Source: CAD feature listing. Evaluate the final solid. Frame: model axes, mm. Face numbers are marked on the shaded views. A direction names the side the tool comes from. Give positions to 0.01 mm unless a question says otherwise; leave off trailing zeros. Loops run counter-clockwise (first coordinate to the right, second up) from the corner with the lowest first, then second, coordinate; pieces in that order, holes last. Notation, with made-up numbers: (34.25, 76) -> (61.25, 76) arc R23 cw to (61.25, 113) -> close; hole circle Ø3 at (-30.75, 31). An arc over 180 degrees is marked (long way). Put each result on its own line as item: value.
```python
from build123d import *

# Parameters (mm, degrees)
SKETCH1_R               = 17.5
SKETCH1_R_2             = 12.5
BOSS_EXTRUDE1_DEPTH     = 152.4
SKETCH2_R               = 19.05
SKETCH2_R_2             = 17.5
BOSS_EXTRUDE2_DEPTH     = 8
SKETCH4_R               = 17.5
SKETCH4_R_2             = 16
CUT_EXTRUDE2_DEPTH      = 2
FILLET1_R               = 0.4064
CUT_EXTRUDE3_DEPTH      = 155.762931608
CUT_EXTRUDE3_DEPTH_BACK = 155.762931608
SKETCH8_W               = 25.4
SKETCH8_H               = 3.175
FILLET2_R               = 3.175
CUT_EXTRUDE4_REACH      = 156.763
CUT_EXTRUDE4_END_RADIUS = 17.5


with BuildPart() as part:
    # Sketch1 → Boss-Extrude1 (new, symmetric)
    with BuildSketch(Plane(origin=(0, 0, 0), x_dir=(0, 0, -1), z_dir=(1, 0, 0))):
        with Locations(Location((0, 0, 0), (0, 0, 180))):
            Circle(SKETCH1_R)
        with Locations(Location((0, 0, 0), (0, 0, 180))):
            Circle(SKETCH1_R_2, mode=Mode.SUBTRACT)
    extrude(amount=BOSS_EXTRUDE1_DEPTH, both=True)

    # Sketch2 → Boss-Extrude2 (add)
    with BuildSketch(Plane.ZY.offset(-92.4)):
        Circle(SKETCH2_R)
        Circle(SKETCH2_R_2, mode=Mode.SUBTRACT)
    extrude(amount=BOSS_EXTRUDE2_DEPTH)

    # Sketch4 → Cut-Extrude2 (cut)
    with BuildSketch(Plane(origin=(133.52, 0, 0), x_dir=(0, 0, -1), z_dir=(1, 0, 0))):
        with Locations(Location((0, 0, 0), (0, 0, 180))):
            Circle(SKETCH4_R)
        Circle(SKETCH4_R_2, mode=Mode.SUBTRACT)
    extrude(amount=-CUT_EXTRUDE2_DEPTH, mode=Mode.SUBTRACT)

    # Fillet1
    fillet1_edges = [part.edges().sort_by_distance(p)[0] for p in [
        (131.52, 0, 16),
        (133.52, 0, 16),
    ]]
    fillet(fillet1_edges, radius=FILLET1_R)

    # Sketch8 → Cut-Extrude3 (cut, two sides: drawn at the far end of the back side and taken through both)
    with BuildSketch(Plane.XY.offset(-CUT_EXTRUDE3_DEPTH_BACK)):
        with Locations((36.7, 17.4625)):
            Rectangle(SKETCH8_W, SKETCH8_H)
        with Locations((36.7, -17.4625)):
            Rectangle(SKETCH8_W, SKETCH8_H)
    extrude(amount=CUT_EXTRUDE3_DEPTH + CUT_EXTRUDE3_DEPTH_BACK, mode=Mode.SUBTRACT)

    # Fillet2
    # the kernel refuses this fillet: 3.175 mm, written as the material it adds along each edge
    with BuildSketch(Plane(origin=(49.4, -15.875, 15.301899161), x_dir=(-1, 0, 0), z_dir=(0, 0, -1))) as fillet2_piece_1_section:
        with BuildLine():
            CenterArc((FILLET2_R, -FILLET2_R), FILLET2_R, 90, 90)
            Line((0, -FILLET2_R), (0, 0))
            Line((0, 0), (FILLET2_R, 0))
        make_face()
    fillet2_piece_1 = extrude(amount=30.603798322, mode=Mode.PRIVATE)
    fillet2_piece_1 = fillet2_piece_1 & Plane(origin=(48.505622485, 0, 0), x_dir=(0, 0, 1), z_dir=(1, 0, 0)) * Cylinder(17.5, 74, mode=Mode.PRIVATE)
    add(fillet2_piece_1)
    with BuildSketch(Plane(origin=(24, -15.875, -15.301899161), x_dir=(1, 0, 0), z_dir=(0, 0, 1))) as fillet2_piece_2_section:
        with BuildLine():
            CenterArc((FILLET2_R, -FILLET2_R), FILLET2_R, 90, 90)
            Line((0, -FILLET2_R), (0, 0))
            Line((0, 0), (FILLET2_R, 0))
        make_face()
    fillet2_piece_2 = extrude(amount=30.603798322, mode=Mode.PRIVATE)
    fillet2_piece_2 = fillet2_piece_2 & Plane(origin=(24.894377515, 0, 0), x_dir=(0, 0, 1), z_dir=(1, 0, 0)) * Cylinder(17.5, 74, mode=Mode.PRIVATE)
    add(fillet2_piece_2)
    with BuildSketch(Plane(origin=(49.4, 15.875, 15.301899161), x_dir=(-1, 0, 0), z_dir=(0, 0, -1))) as fillet2_piece_3_section:
        with BuildLine():
            CenterArc((FILLET2_R, FILLET2_R), FILLET2_R, 180, 90)
            Line((0, FILLET2_R), (0, 0))
            Line((0, 0), (FILLET2_R, 0))
        make_face()
    fillet2_piece_3 = extrude(amount=30.603798322, mode=Mode.PRIVATE)
    fillet2_piece_3 = fillet2_piece_3 & Plane(origin=(48.50564536, 0, 0), x_dir=(0, 0, 1), z_dir=(1, 0, 0)) * Cylinder(17.5, 74, mode=Mode.PRIVATE)
    add(fillet2_piece_3)
    with BuildSketch(Plane(origin=(24, 15.875, -15.301899161), x_dir=(0, 1, 0), z_dir=(0, 0, 1))) as fillet2_piece_4_section:
        with BuildLine():
            CenterArc((FILLET2_R, -FILLET2_R), FILLET2_R, 90, 90)
            Line((0, -FILLET2_R), (0, 0))
            Line((0, 0), (FILLET2_R, 0))
        make_face()
    fillet2_piece_4 = extrude(amount=30.603798322, mode=Mode.PRIVATE)
    fillet2_piece_4 = fillet2_piece_4 & Plane(origin=(24.89438719, 0, 0), x_dir=(0, 0, 1), z_dir=(1, 0, 0)) * Cylinder(17.5, 74, mode=Mode.PRIVATE)
    add(fillet2_piece_4)

    # Cut-Extrude4: up to this cylinder (the profile starts inside it)
    cut_extrude4_end = Plane(origin=(36.7, 0, 0), z_dir=(-1, 0, 0)) * Cylinder(CUT_EXTRUDE4_END_RADIUS, 349.526, mode=Mode.PRIVATE)
    # Sketch9 → Cut-Extrude4 (cut, up to the surface)
    with BuildSketch(Plane.XY, mode=Mode.PRIVATE) as cut_extrude4_sk1:
        with BuildLine():
            Line((43.05, -6.35), (30.35, -6.35))
            ThreePointArc((30.35, -6.35), (24, 0), (30.35, 6.35))
            Line((30.35, 6.35), (43.05, 6.35))
            ThreePointArc((43.05, 6.35), (49.4, 0), (43.05, -6.35))
        make_face()
    cut_extrude4_tool1 = extrude(cut_extrude4_sk1.sketch, amount=CUT_EXTRUDE4_REACH, mode=Mode.PRIVATE) & cut_extrude4_end
    add(cut_extrude4_tool1.solids().sort_by_distance((36.7, 0, 0))[0], mode=Mode.SUBTRACT)


solid = part.part
```
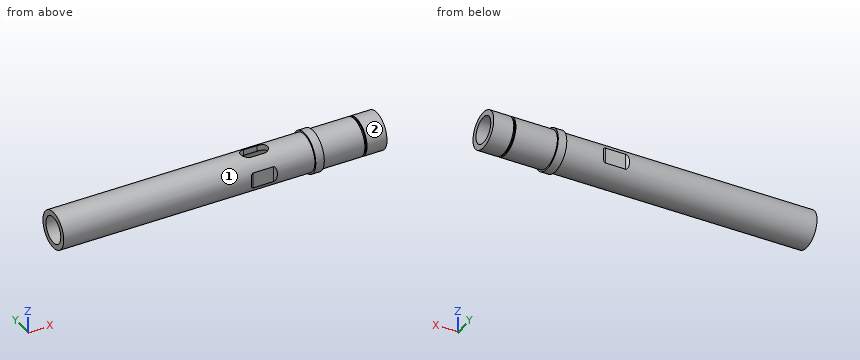
(1) Reachability of the marked faces 1 and 2 from +Z, -Z, +X, -X, +Y, -Y: full face, straight path, thin tool, end or side. Return the list, or none.
Calculated:
face 1: -X
face 2: +X
(2) First-contact query: P1, Ø4, axis at x = 81.5, y = 15, coming from the -Z side; P2, Ø4.5, axis at x = 36, z = -3.5, coming from the +Y side (3 decimals); P3, Ø10, axis at x = 96, z = -2, coming from the +Y side; P4, Ø15, axis at y = 0, z = 0, coming from the +X side. Flat tips, straight axial feed; report the tip coordinate or a pass-through.
Calculated:
P1: stops at z = -11.72
P2: stops at y = 15.875
P3: stops at y = 19.05
P4: passes through
(3) Line query: probe 1 along Y at (x, z) = (-57.5, 0); probe 2 along Z at (x, y) = (35, 0); probe 3 along Z at (x, y) = (-31.5, 5). Output: solid intervals per line, ascending. Write a range as from..to.
Calculated:
probe 1: y = -17.5..-12.5, 12.5..17.5
probe 2: z = -17.5..-12.5
probe 3: z = -16.77..-11.46, 11.46..16.77
(4) Section A-A on y = 0. Give the number of separate pieces and of enclosed holes in the cut face, then the cut area to 3 significant figures.
Calculated:
separate pieces: 3
enclosed holes: 0
area: 2,940 mm²
(5) Section B-B on x = 126. Return loops of the section in (y, z).
Calculated:
outline: circle Ø35 at (0, 0); hole circle Ø25 at (0, 0)
